```python
from build123d import *

# Parameters (mm, degrees)
SKETCH1_R                       = 57.15
BOSS_EXTRUDE1_DEPTH             = 63.5
SKETCH2_R                       = 41.275
CUT_EXTRUDE1_DEPTH              = 53.34
F_1_4_0_25_DIAMETER_HOLE4_D     = 6.35
F_1_4_0_25_DIAMETER_HOLE4_DEPTH = 25.4
F_1_4_0_25_DIAMETER_HOLE4_TIP   = 1.907732465
SKETCH7_R                       = 3.81
CUT_EXTRUDE2_DEPTH              = 103.783729257
F_4_0MM_DOWEL_HOLE1_D           = 4
SKETCH9_W                       = 7
SKETCH9_H                       = 7
CUT_EXTRUDE3_DEPTH              = 3.5
SKETCH12_W                      = 12.7
SKETCH12_H                      = 19.05
CUT_EXTRUDE4_DEPTH              = 4.7625
SKETCH13_R                      = 64.794556677
CUT_EXTRUDE5_DEPTH              = 59.69


with BuildPart() as part:
    # Sketch1 → Boss-Extrude1 (new body)
    with BuildSketch(Plane(origin=(0, 0, 0), x_dir=(1, 0, 0), z_dir=(0, 1, 0))):
        with Locations(Location((0, 0, 0), (0, 0, 270))):
            Circle(SKETCH1_R)
    extrude(amount=BOSS_EXTRUDE1_DEPTH)

    # Sketch2 → Cut-Extrude1 (cut)
    with BuildSketch(Plane(origin=(0, 63.5, 0), x_dir=(1, 0, 0), z_dir=(0, 1, 0))):
        with Locations(Location((0, 0, 0), (0, 0, 270))):
            Circle(SKETCH2_R)
    extrude(amount=-CUT_EXTRUDE1_DEPTH, mode=Mode.SUBTRACT)

    # 1/4 (0.25) Diameter Hole4
    with Locations(Plane(origin=(0, 63.5, 0), x_dir=(1, 0, 0), z_dir=(0, 1, 0))):
        with Locations((-41.244459855, 23.8125), (0, -47.625), (41.244459855, 23.8125)):
            Hole(F_1_4_0_25_DIAMETER_HOLE4_D / 2, depth=F_1_4_0_25_DIAMETER_HOLE4_DEPTH)
            with Locations((0, 0, -(F_1_4_0_25_DIAMETER_HOLE4_DEPTH + F_1_4_0_25_DIAMETER_HOLE4_TIP / 2))):  # 118° drill point
                Cone(0, F_1_4_0_25_DIAMETER_HOLE4_D / 2, F_1_4_0_25_DIAMETER_HOLE4_TIP, mode=Mode.SUBTRACT)

    # Sketch7 → Cut-Extrude2 (cut, through all)
    with BuildSketch(Plane.XY):
        with Locations((0, 15.24)):
            Circle(SKETCH7_R)
    extrude(amount=-CUT_EXTRUDE2_DEPTH, mode=Mode.SUBTRACT)

    # Ø4.0mm Dowel Hole1 (through all)
    with Locations(Plane(origin=(-5, 0, 15.938504039), x_dir=(0, 0, -1), z_dir=(0, -1, 0))):
        with Locations((0, 0), (0, 10), (49.5, 10), (49.5, 0)):
            Hole(F_4_0MM_DOWEL_HOLE1_D / 2)

    # Sketch9 → Cut-Extrude3 (cut)
    with BuildSketch(Plane.XZ):
        with Locations((-5, 15.938504039)):
            Rectangle(SKETCH9_W, SKETCH9_H)
        with Locations((5, 15.938504039)):
            Rectangle(SKETCH9_W, SKETCH9_H)
        with Locations((5, -33.561495961)):
            Rectangle(SKETCH9_W, SKETCH9_H)
        with Locations((-5, -33.561495961)):
            Rectangle(SKETCH9_W, SKETCH9_H)
    extrude(amount=-CUT_EXTRUDE3_DEPTH, mode=Mode.SUBTRACT)

    # Sketch12 → Cut-Extrude4 (cut)
    with BuildSketch(Plane(origin=(0, 50.8, 0), x_dir=(1, 0, 0), z_dir=(0, 1, 0))):
        Polygon((-54.992429237, 24.417545405), (-38.494645295, 14.892545405), (-35.319645295, 20.391806719), (-51.817429237, 29.916806719), align=None)
        Polygon((-51.817429237, 29.916806719), (-35.319645295, 20.391806719), (-32.144645295, 25.891068033), (-48.642429237, 35.416068033), align=None)
        Polygon((32.144645295, 25.891068033), (35.319645295, 20.391806719), (51.817429237, 29.916806719), (48.642429237, 35.416068033), align=None)
        Polygon((51.817429237, 29.916806719), (35.319645295, 20.391806719), (38.494645295, 14.892545405), (54.992429237, 24.417545405), align=None)
        with Locations((0, -50.308613437)):
            Rectangle(SKETCH12_W, SKETCH12_H)
    extrude(amount=CUT_EXTRUDE4_DEPTH, mode=Mode.SUBTRACT)

    # Sketch13 → Cut-Extrude5 (cut)
    with BuildSketch(Plane.XZ):
        Circle(SKETCH13_R)
    extrude(amount=-CUT_EXTRUDE5_DEPTH, mode=Mode.SUBTRACT)


solid = part.part
```
Check sheet for the modelled part. Datum: model origin and axes. Units: mm. Round coordinates to 2 decimals unless told otherwise and drop trailing zeros. Order: outer loops, then holes, each group sorted by start corner. A loop starts at its lowest first (then second) coordinate and runs counter-clockwise, first axis right, second up. Notation, with made-up numbers: (35, 82.25) - (62, 82.25) arc R19 ccw to (62, 103.25) - close; hole circle Ø8 at (-40, -13.5). An arc over 180 degrees is marked (long way). Answer as CSV lines item,"result". Start each with the question number.
1) Depth check by flat-ended pin: pin 1 (8.5 mm diameter, centred on x = 41.24, z = -23.81, fed in from -Y); pin 2 (2 mm diameter, centred on y = 61.5, z = 14.5, fed in from -X); pin 3 (10 mm diameter, centred on x = 15.5, z = -29.5, fed in from -Y) (1 decimal); pin 4 (1.5 mm diameter, centred on y = 62, z = 25, fed in from +X). Enter the tip coordinate at first touch or a pass-through.
2) Section check D-D (y = 62.6). Give the number of separate pieces and of enclosed holes in the cut face, then the cut area to 3 significant figures.
3) Section check C-C (x = -15.5). Record the cut outline in (y, z).
4) Draft check along X on faces 1 (the face through (17, 59.69, -38)), 2 (the face through (2.513, 61.568, -57.095)), 3 (the face through (-44.18, 61.57, -22.6)), 4 (the face through (0.688, 61.568, 50.724)). Enter one of: +X half, -X half, draft (parallel to the pull), parting line (faces both ways), or undercut.
5) Section check A-A (z = 0). Record the cut outline in (x, y) (3 decimals).
6) Scan lines: probe 1 along X at (y, z) = (62.7, 0) (3 decimals); probe 2 along Z at (x, y) = (-29, 62.1); probe 3 along X at (y, z) = (60.9, -5). Record each from-to range of solid material in increasing order.
7) Section check B-B (x = 0). Record the cut outline in (y, z) (3 decimals), then the cut area to 3 significant figures.
Determined:
1,pin 1,"y = 59.69"
1,pin 2,"x = -55.53"
1,pin 3,"through"
1,pin 4,"x = 51.75"
2,separate pieces,"1"
2,enclosed holes,"4"
2,area,"4,810 mm^2"
3,outline,"(59.69, -55.01) - (63.5, -55.01) - (63.5, -38.25) - (59.69, -38.25) - close; (59.69, 38.25) - (63.5, 38.25) - (63.5, 55.01) - (59.69, 55.01) - close"
4,face 1,"draft"
4,face 2,"parting line"
4,face 3,"undercut"
4,face 4,"undercut"
5,outline,"(-57.15, 59.69) - (-41.275, 59.69) - (-41.275, 63.5) - (-57.15, 63.5) - close; (41.275, 59.69) - (57.15, 59.69) - (57.15, 63.5) - (41.275, 63.5) - close"
6,probe 1,"-57.15 to -41.275, 41.275 to 57.15"
6,probe 2,"-49.25 to -29.37, 29.37 to 49.25"
6,probe 3,"-56.93 to -40.97, 40.97 to 56.93"
7,outline,"(59.69, -57.15) - (63.5, -57.15) - (63.5, -41.275) - (59.69, -41.275) - close; (59.69, 41.275) - (63.5, 41.275) - (63.5, 44.45) - (59.69, 44.45) - close; (59.69, 50.8) - (63.5, 50.8) - (63.5, 57.15) - (59.69, 57.15) - close"
7,area,"96.8 mm^2"
